from build123d import *

# Parameters (mm, degrees)
BOSS_EXTRUDE1_DEPTH     = 12
CUT_EXTRUDE1_DEPTH      = 10
FILLET1_R               = 4
BOSS_EXTRUDE3_DEPTH     = 1
MIRROR2_COPY_1_DEPTH    = 1
SKETCH3_W               = 14.5
SKETCH3_H               = 5.622498999
CUT_EXTRUDE2_DEPTH      = 2
CUT_EXTRUDE2_DEPTH_BACK = 8
SKETCH4_W               = 4.5
SKETCH4_H               = 4.973684211
CUT_EXTRUDE3_DEPTH      = 3


with BuildPart() as part:
    # Sketch1 → Boss-Extrude1 (new body)
    with BuildSketch(Plane(origin=(0, 0, 0), x_dir=(1, 0, 0), z_dir=(0, 1, 0))):
        with BuildLine():
            Line((-8, -13), (8, -13))
            ThreePointArc((8, -13), (14.828427125, -15.828427125), (12, -9))
            Line((12, -9), (12, 9))
            ThreePointArc((12, 9), (14.828427125, 15.828427125), (8, 13))
            Line((8, 13), (-8, 13))
            ThreePointArc((-8, 13), (-14.828427125, 15.828427125), (-12, 9))
            Line((-12, 9), (-12, -9))
            ThreePointArc((-12, -9), (-14.828427125, -15.828427125), (-8, -13))
        make_face()
    extrude(amount=BOSS_EXTRUDE1_DEPTH)

    # Sketch2 → Cut-Extrude1 (cut)
    with BuildSketch(Plane(origin=(0, 12, 0), x_dir=(1, 0, 0), z_dir=(0, 1, 0))):
        Polygon((-9.5, -10.5), (5, -10.5), (5, -5.526315789), (9.5, -5.526315789), (9.5, 10.5), (-5, 10.5), (-5, 5.526315789), (-9.5, 5.526315789), align=None)
    extrude(amount=-CUT_EXTRUDE1_DEPTH, mode=Mode.SUBTRACT)

    # Fillet1
    fillet1_edges = [part.edges().sort_by_distance(p)[0] for p in [
        (12, 6, -9),
        (12, 6, 9),
        (8, 6, 13),
        (-8, 6, 13),
        (-12, 6, 9),
        (-12, 6, -9),
        (-8, 6, -13),
        (8, 6, -13),
    ]]
    fillet(fillet1_edges, radius=FILLET1_R)

    # Sketch10 → Boss-Extrude3 (add)
    with BuildSketch(Plane(origin=(0, 12, 0), x_dir=(1, 0, 0), z_dir=(0, 1, 0))):
        with BuildLine():
            Line((14.417326185, -9.813068229), (14.165063509, -10.25))
            ThreePointArc((14.165063509, -10.25), (9.525126266, -10.525126266), (9.25, -15.165063509))
            Line((9.25, -15.165063509), (8.813068229, -15.417326185))
            ThreePointArc((8.813068229, -15.417326185), (14.828427125, -15.828427125), (14.417326185, -9.813068229))
        make_face()
    boss_extrude3 = extrude(amount=BOSS_EXTRUDE3_DEPTH)

    # Mirror1: Boss-Extrude3 across plane
    add(boss_extrude3.mirror(Plane(origin=(0, 0, 0), x_dir=(0, 0, 1), z_dir=(1, 0, 0))))

    # Mirror2: Boss-Extrude3 across plane
    add(boss_extrude3.mirror(Plane.XY))

    # Mirror2 copy 1 sketch → Mirror2 copy 1 (add)
    with BuildSketch(Plane(origin=(0, 12, 0), x_dir=(-1, 0, 0), z_dir=(0, 1, 0))):
        with BuildLine():
            Line((14.417326185, -9.813068229), (14.165063509, -10.25))
            ThreePointArc((14.165063509, -10.25), (9.525126266, -10.525126266), (9.25, -15.165063509))
            Line((9.25, -15.165063509), (8.813068229, -15.417326185))
            ThreePointArc((8.813068229, -15.417326185), (14.828427125, -15.828427125), (14.417326185, -9.813068229))
        make_face()
    extrude(amount=MIRROR2_COPY_1_DEPTH)

    # Sketch3 → Cut-Extrude2 (cut, two sides)
    with BuildSketch(Plane(origin=(0, 12, 0), x_dir=(1, 0, 0), z_dir=(0, 1, 0))) as cut_extrude2_sk:
        with Locations((-2.25, -13.3112495)):
            Rectangle(SKETCH3_W, SKETCH3_H)
    extrude(amount=CUT_EXTRUDE2_DEPTH, mode=Mode.SUBTRACT)
    extrude(cut_extrude2_sk.sketch, amount=-CUT_EXTRUDE2_DEPTH_BACK, mode=Mode.SUBTRACT)

    # Sketch4 → Cut-Extrude3 (cut)
    with BuildSketch(Plane(origin=(0, 12, 0), x_dir=(1, 0, 0), z_dir=(0, 1, 0))):
        with Locations((-7.25, 8.013157895)):
            Rectangle(SKETCH4_W, SKETCH4_H)
        with Locations((7.25, -8.013157895)):
            Rectangle(SKETCH4_W, SKETCH4_H)
    extrude(amount=-CUT_EXTRUDE3_DEPTH, mode=Mode.SUBTRACT)


solid = part.part
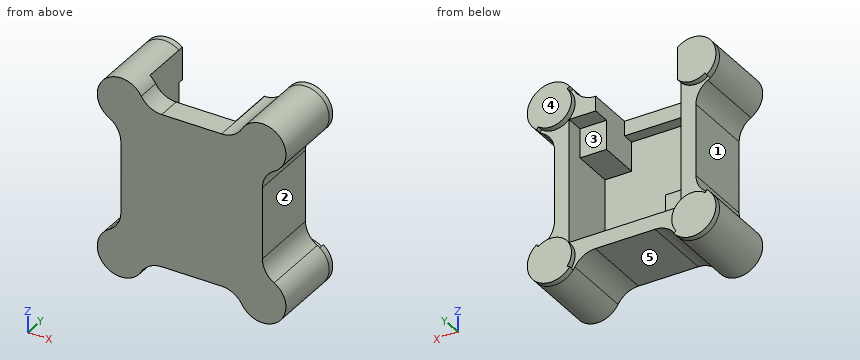
Could you check a few things on this model? Use its own coordinates, in mm. Face numbers are marked on the shaded views. A direction names the side the tool comes from. Give positions to 0.01 mm unless a question says otherwise; leave off trailing zeros. Loops run counter-clockwise (first coordinate to the right, second up) from the corner with the lowest first, then second, coordinate; pieces in that order, holes last. Notation, with made-up numbers: (19.25, 16.25) -> (34.25, 16.25) arc R17 ccw to (34.25, 32.25) -> close; hole circle Ø6 at (-1, 10). An arc over 180 degrees is marked (long way). Return JSON: item names as keys, results as strings.
Item 1: If we section it at C-C on x = -3.5: List the corners of the cut face in (y, z) for me, plus the area to 3 significant figures.
Geometry results:
{"outline": "(0, -13) -> (12, -13) -> (12, -10.5) -> (2, -10.5) -> (2, 10.5) -> (4, 10.5) -> (4, 13) -> (0, 13) -> close", "area": "82.0 mm²"}
Item 2: I'm going to push flat-ended pins straight in: pin 1 (2 mm diameter, centred on x = 8, y = 5, fed in from -Z); pin 2 (14.5 mm diameter, centred on x = -1, z = 6, fed in from +Y); pin 3 (5 mm diameter, centred on x = 3.5, y = 7.5, fed in from +Z). Where does each tip first touch, or does it pass through?
Geometry results:
{"pin 1": "stops at z = -15.65", "pin 2": "stops at y = 9", "pin 3": "stops at z = 13.11"}
Item 3: Which directions (+Z, -Z, +X, -X, +Y, -Y) give clear straight access to the entire face, cutting with the end or side of a thin tool? Please do the marked faces 1, 2, 3, 4 and 5.
Geometry results:
{"face 1": "-X, +Y, -Y", "face 2": "+X, +Y, -Y", "face 3": "+Y", "face 4": "+Z, -Z, +X, -X, +Y", "face 5": "-Z, +Y, -Y"}
Item 4: If we section it at B-B on z = 5: List the corners of the cut face in (x, y) for me, plus the area to 3 significant figures.
Geometry results:
{"outline": "(-12, 0) -> (12, 0) -> (12, 12) -> (9.5, 12) -> (9.5, 2) -> (-9.5, 2) -> (-9.5, 12) -> (-12, 12) -> close", "area": "98.0 mm²"}
Item 5: I need wall thicknesses on L1, parallel to X at y = 5.5, z = 4; L2, parallel to Z at x = 6, y = 2.75; L3, parallel to Y at x = 7, z = 13. Which ranges of each line are inside material? Lowest first, please. Write a range as from..to.
Geometry results:
{"L1": "x = -12..-9.5, 9.5..12", "L2": "z = -13.11..-10.5, 5.53..13.11", "L3": "y = 0..12"}
Item 6: If we section it at A-A on y = 2.75: List the corners of the cut face in (x, z) for me, plus the area to 3 significant figures.
Geometry results:
{"outline": "(-14, -9.54) arc R4 ccw (long way) to (-8.54, -15) arc R4 cw to (-5.07, -13) -> (5.07, -13) arc R4 cw to (8.54, -15) arc R4 ccw (long way) to (14, -9.54) arc R4 cw to (12, -6.07) -> (12, 6.07) arc R4 cw to (14, 9.54) arc R4 ccw (long way) to (8.54, 15) arc R4 cw to (5.07, 13) -> (-5.07, 13) arc R4 cw to (-8.54, 15) arc R4 ccw (long way) to (-14, 9.54) arc R4 cw to (-12, 6.07) -> (-12, -6.07) arc R4 cw to start; hole (-9.5, -5.53) -> (-5, -5.53) -> (-5, -10.5) -> (9.5, -10.5) -> (9.5, 5.53) -> (5, 5.53) -> (5, 10.5) -> (-9.5, 10.5) -> close", "area": "431 mm²"}
Item 7: If we section it at D-D on y = 11: List the corners of the cut face in (x, z) for me.
Geometry results:
{"outline": "(-14, -9.54) arc R4 ccw (long way) to (-8.54, -15) arc R4 cw to (-5.07, -13) -> (5.07, -13) arc R4 cw to (8.54, -15) arc R4 ccw (long way) to (14, -9.54) arc R4 cw to (12, -6.07) -> (12, 6.07) arc R4 cw to (14, 9.54) arc R4 ccw (long way) to (8.54, 15) arc R4 cw to (5.07, 13) -> (5, 13) -> (5, 10.5) -> (9.5, 10.5) -> (9.5, -10.5) -> (-9.5, -10.5) -> (-9.5, 16.12) arc R4 ccw (long way) to (-14, 9.54) arc R4 cw to (-12, 6.07) -> (-12, -6.07) arc R4 cw to start"}
